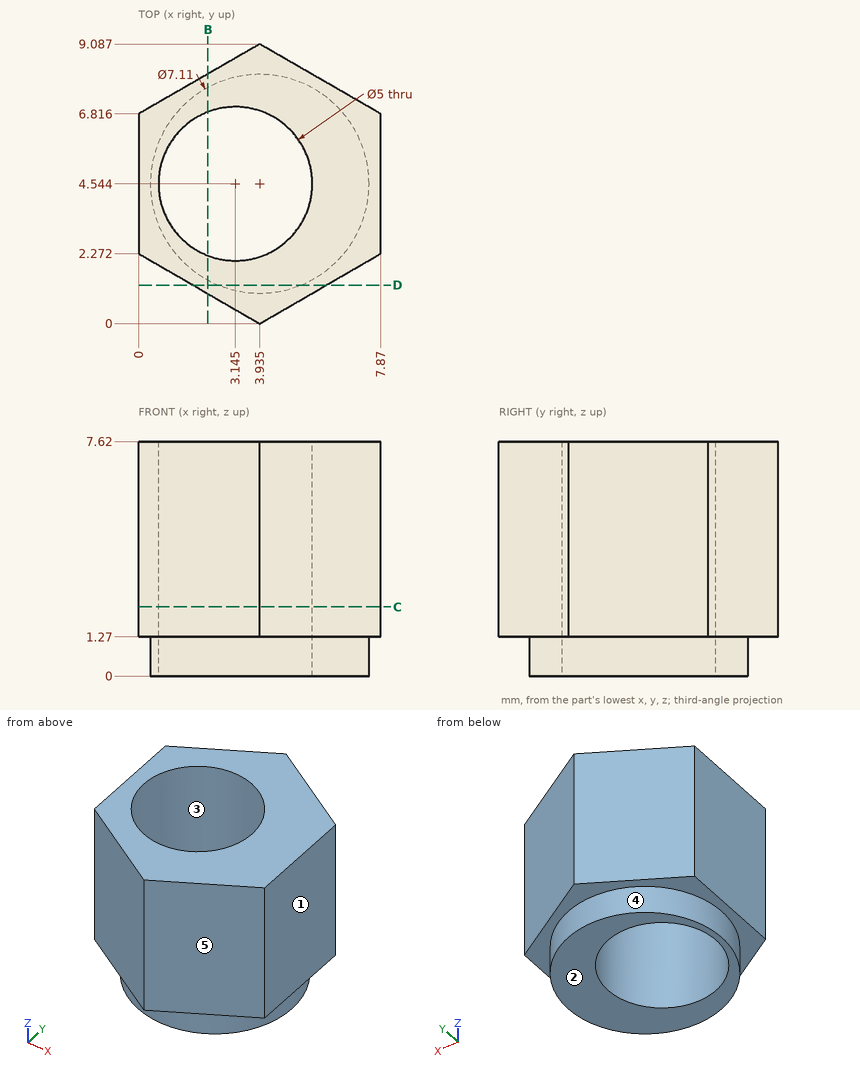
The drawing under review shows one solid part. Ordinate dimensions are in mm from its lowest x, y, z. A direction names the side the tool comes from. Round coordinates to 2 decimals unless told otherwise and drop trailing zeros. Order: outer loops, then holes, each group sorted by start corner. A loop starts at its lowest first (then second) coordinate and runs counter-clockwise, first axis right, second up. Notation, with made-up numbers: (9, -16.5) -> (33, -16.5) arc R24 ccw to (33, 21.5) -> close; hole circle Ø6 at (63.25, 44). An arc over 180 degrees is marked (long way). Return JSON: item names as keys, results as strings.
1. For the marked faces 4 and 5, list the 3-axis set-ups (+Z, -Z, +X, -X, +Y, -Y) from which the entire face can be reached by the end or side of a thin tool; tool diameter is ignored.
Answer block:
{"face 4": "-Z", "face 5": "+Z, -Z, +X, -Y"}
2. Insertion check: P1, Ø4, axis at x = 3, y = 3, coming from the -Z side; P2, Ø4, axis at x = 1, z = 5, coming from the +Y side. Each pin has a flat end and moves straight along its axis. Give the tip position at first contact, or say it passes through.
Answer block:
{"P1": "stops at z = 0", "P2": "stops at y = 8.55"}
3. The part is to be moulded in two halves that separate along X. For the marked faces 1, 2 and 3, say which applies: +X half, -X half, draft (parallel to the pull), parting line (faces both ways), or undercut.
Answer block:
{"face 1": "+X half", "face 2": "draft", "face 3": "undercut"}
4. Take a section at D-D (y = 1.25). Write out the cut boundary in (x, z), then the cut area to 3 significant figures.
Answer block:
{"outline": "(1.77, 1.27) -> (2.6, 1.27) -> (2.6, 0) -> (5.27, 0) -> (5.27, 1.27) -> (6.1, 1.27) -> (6.1, 7.62) -> (1.77, 7.62) -> close", "area": "30.9 mm²"}
5. For L1, parallel to Z at x = 7.5, y = 3; L2, parallel to X at y = 3.5, z = 5.5 (1 decimal); L3, parallel to X at y = 6.5, z = 1 (1 decimal), list the stretches that pass through material, from the lowest coordinate up. Write a range as [from, to].
Answer block:
{"L1": "z = [1.27, 7.62]", "L2": "x = [0, 0.9], [5.4, 7.9]", "L3": "x = [1, 1.6], [4.7, 6.9]"}
6. Take a section at B-B (x = 2.25). Write out the cut boundary in (y, z) (1 decimal).
Answer block:
{"outline": "(1, 1.3) -> (1.4, 1.3) -> (1.4, 0) -> (2.2, 0) -> (2.2, 7.6) -> (1, 7.6) -> close; (6.9, 0) -> (7.7, 0) -> (7.7, 1.3) -> (8.1, 1.3) -> (8.1, 7.6) -> (6.9, 7.6) -> close"}
7. Take a section at C-C (z = 2.25). Write out the cut boundary in (x, y) (1 decimal).
Answer block:
{"outline": "(0, 2.3) -> (3.9, 0) -> (7.9, 2.3) -> (7.9, 6.8) -> (3.9, 9.1) -> (0, 6.8) -> close; hole circle Ø5 at (3.1, 4.5)"}
